Here's how the part is built. I have some questions about the finished solid (model axes, mm). Face numbers are marked on the shaded views. A direction names the side the tool comes from. Coordinates: 2 decimals unless noted, no trailing zeros. Write each loop counter-clockwise with the first axis right and the second up, starting at its lowest first coordinate (ties: lowest second). Pieces come first, ordered by that corner, then holes.
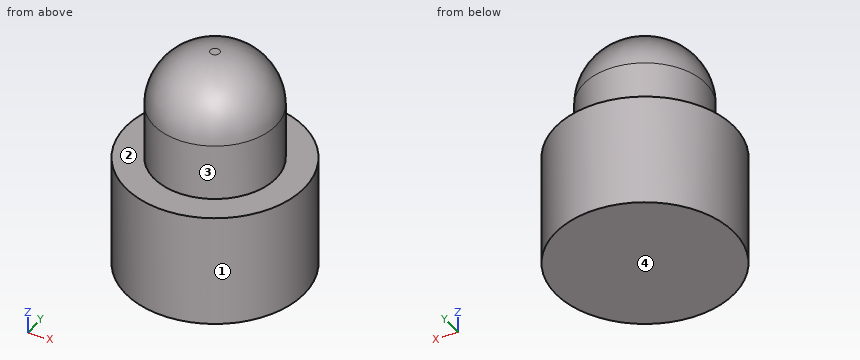
```python
from build123d import *

# Parameters (mm, degrees)
F0_R     = 3.25
F1_DEPTH = 12
F0_R_2   = 4.75
F2_DEPTH = 6
F3_R     = 3


with BuildPart() as f1:
    # F0 (on Top) → F1 (new body)
    with BuildSketch(Plane.XY):
        Circle(F0_R)
    extrude(amount=F1_DEPTH)

    # F0 (on Top) → F2 (join)
    with BuildSketch(Plane.XY):
        Circle(F0_R_2)
        Circle(F0_R, mode=Mode.SUBTRACT)
    extrude(amount=F2_DEPTH)

    # F3
    f3_edges = [f1.edges().sort_by_distance(p)[0] for p in [
        (-3.25, 0, 12),
    ]]
    fillet(f3_edges, radius=F3_R)


solid = f1.part
```
1) Imagine slicing it at A-A on z = 1.5. Please give me the cut outline in (x, y).
Values follow:
outline: circle Ø9.5 at (0, 0)
2) Imagine slicing it at C-C on y = 4.25. Please give me the cut outline in (x, z).
Values follow:
outline: (-2.12, 0) - (2.12, 0) - (2.12, 6) - (-2.12, 6) - close
3) Will these pins go through, and if not, where does the flat tip stop? pin 1 (3 mm diameter, centred on x = 2, y = 0.5, fed in from +Z); pin 2 (4 mm diameter, centred on x = 0, y = 3, fed in from -Z); pin 3 (1 mm diameter, centred on y = -0.5, z = 7, fed in from +X); pin 4 (1.5 mm diameter, centred on x = 2.5, z = 9, fed in from -Y).
Values follow:
pin 1: stops at z = 11.98
pin 2: stops at z = 0
pin 3: stops at x = 3.25
pin 4: stops at y = -2.74
4) Imagine slicing it at D-D on z = 8.25. Please give me the cut outline in (x, y).
Values follow:
outline: circle Ø6.5 at (0, 0)
5) Imagine slicing it at B-B on x = 3.5. Please give me the cut outline in (y, z).
Values follow:
outline: (-3.21, 0) - (3.21, 0) - (3.21, 6) - (-3.21, 6) - close
6) On a 3-axis mill with a long thin cutter (end or side, diameter ignored), from which of +Z, -Z, +X, -X, +Y, -Y can I reach the whole of each face in a straight line? I mean the marked faces 1 and 2. Say none if no direction works.
Values follow:
face 1: +Z, -Z
face 2: +Z
7) I need wall thicknesses on probe 1 along Z at (x, y) = (-2.5, -2.25); probe 2 along Z at (x, y) = (0, -1.5); probe 3 along X at (y, z) = (0.25, 2). Which ranges of each line are inside material? Lowest first, please.
Values follow:
probe 1: z = 0 to 6
probe 2: z = 0 to 11.73
probe 3: x = -4.74 to 4.74
8) We'd pull the mould along X, two halves only. Please class the marked faces 3 and 4: pulls with the +X half, pulls with the -X half, needs draft (parallel to the pull), parting line crosses it, or undercut.
Values follow:
face 3: parting line crosses it
face 4: needs draft
